```python
from build123d import *

# Parameters (mm, degrees)
SKETCH1_R           = 16
SKETCH1_R_2         = 12
BOSS_EXTRUDE1_DEPTH = 18
SKETCH1_3_R         = 3
BOSS_EXTRUDE2_DEPTH = 5
BOSS_EXTRUDE4_DEPTH = 18
SKETCH18_W          = 13
SKETCH18_H          = 2.498753947


with BuildPart() as part:
    # Sketch1 → Boss-Extrude1 (new body)
    with BuildSketch(Plane(origin=(0, 0, 0), x_dir=(1, 0, 0), z_dir=(0, 1, 0))):
        with Locations(Location((0, 0, 0), (0, 0, 270))):
            Circle(SKETCH1_R)
        with Locations(Location((0, 0, 0), (0, 0, 270))):
            Circle(SKETCH1_R_2, mode=Mode.SUBTRACT)
    extrude(amount=BOSS_EXTRUDE1_DEPTH)

    # Sketch1_3 → Boss-Extrude2 (add)
    with BuildSketch(Plane(origin=(0, 0, 0), x_dir=(1, 0, 0), z_dir=(0, 1, 0))):
        with BuildLine():
            ThreePointArc((-60, 32), (-64.242640687, 30.242640687), (-66, 26))
            Line((-66, 26), (-66, -26))
            ThreePointArc((-66, -26), (-64.242640687, -30.242640687), (-60, -32))
            Line((-60, -32), (60, -32))
            ThreePointArc((60, -32), (64.242640687, -30.242640687), (66, -26))
            Line((66, -26), (66, 26))
            ThreePointArc((66, 26), (64.242640687, 30.242640687), (60, 32))
            Line((60, 32), (-60, 32))
        make_face()
        with Locations(Location((-60, -26, 0), (0, 0, 270))):
            Circle(SKETCH1_3_R, mode=Mode.SUBTRACT)
        with Locations(Location((60, -26, 0), (0, 0, 270))):
            Circle(SKETCH1_3_R, mode=Mode.SUBTRACT)
        with Locations(Location((-60, 26, 0), (0, 0, 270))):
            Circle(SKETCH1_3_R, mode=Mode.SUBTRACT)
        with BuildLine():
            ThreePointArc((11.047086147, -11.574190583), (0, -16), (-11.047086147, -11.574190583))
            Line((-11.047086147, -11.574190583), (-36.72114317, -26.397114317))
            Line((-36.72114317, -26.397114317), (-41.22114317, -18.602885683))
            Line((-41.22114317, -18.602885683), (-15.547086147, -3.779961949))
            ThreePointArc((-15.547086147, -3.779961949), (-16, 0), (-15.547086147, 3.779961949))
            Line((-15.547086147, 3.779961949), (-41.22114317, 18.602885683))
            Line((-41.22114317, 18.602885683), (-36.72114317, 26.397114317))
            Line((-36.72114317, 26.397114317), (-11.047086147, 11.574190583))
            ThreePointArc((-11.047086147, 11.574190583), (0, 16), (11.047086147, 11.574190583))
            Line((11.047086147, 11.574190583), (36.72114317, 26.397114317))
            Line((36.72114317, 26.397114317), (41.22114317, 18.602885683))
            Line((41.22114317, 18.602885683), (15.547086147, 3.779961949))
            ThreePointArc((15.547086147, 3.779961949), (15.88636803, 1.903499625), (16, 0))
            ThreePointArc((16, 0), (15.88636803, -1.903499625), (15.547086147, -3.779961949))
            Line((15.547086147, -3.779961949), (41.22114317, -18.602885683))
            Line((41.22114317, -18.602885683), (36.72114317, -26.397114317))
            Line((36.72114317, -26.397114317), (11.047086147, -11.574190583))
        make_face(mode=Mode.SUBTRACT)
        with Locations(Location((60, 26, 0), (0, 0, 270))):
            Circle(SKETCH1_3_R, mode=Mode.SUBTRACT)
    extrude(amount=BOSS_EXTRUDE2_DEPTH)

    # Sketch1_6 → Boss-Extrude4 (add)
    with BuildSketch(Plane(origin=(0, 0, 0), x_dir=(1, 0, 0), z_dir=(0, 1, 0))):
        with BuildLine():
            Line((-41.22114317, 18.602885683), (-15.547086147, 3.779961949))
            ThreePointArc((-15.547086147, 3.779961949), (-13.856406461, 8), (-11.047086147, 11.574190583))
            Line((-11.047086147, 11.574190583), (-36.72114317, 26.397114317))
            Line((-36.72114317, 26.397114317), (-41.22114317, 18.602885683))
        make_face()
        with BuildLine():
            Line((36.72114317, 26.397114317), (11.047086147, 11.574190583))
            ThreePointArc((11.047086147, 11.574190583), (13.856406461, 8), (15.547086147, 3.779961949))
            Line((15.547086147, 3.779961949), (41.22114317, 18.602885683))
            Line((41.22114317, 18.602885683), (36.72114317, 26.397114317))
        make_face()
        with BuildLine():
            ThreePointArc((15.547086147, -3.779961949), (13.856406461, -8), (11.047086147, -11.574190583))
            Line((11.047086147, -11.574190583), (36.72114317, -26.397114317))
            Line((36.72114317, -26.397114317), (41.22114317, -18.602885683))
            Line((41.22114317, -18.602885683), (15.547086147, -3.779961949))
        make_face()
        with BuildLine():
            Line((-36.72114317, -26.397114317), (-11.047086147, -11.574190583))
            ThreePointArc((-11.047086147, -11.574190583), (-13.856406461, -8), (-15.547086147, -3.779961949))
            Line((-15.547086147, -3.779961949), (-41.22114317, -18.602885683))
            Line((-41.22114317, -18.602885683), (-36.72114317, -26.397114317))
        make_face()
    extrude(amount=BOSS_EXTRUDE4_DEPTH)

    # Sketch18 → Cut-Revolve4 (revolve, cut)
    with BuildSketch(Plane(origin=(0, 0, 0), x_dir=(0, -1, 0), z_dir=(-1, 0, 0)), mode=Mode.PRIVATE) as cut_revolve4_sk:
        Polygon((-18, 16), (-18, 45), (-5, 45), (-14.422671191, 16), align=None)
        with Locations((-11.5, 46.249376974)):
            Rectangle(SKETCH18_W, SKETCH18_H)
    revolve(cut_revolve4_sk.sketch.rotate(Axis((0, 18.9, 0), (0, -1, 0)), 223.665177219), axis=Axis((0, 18.9, 0), (0, -1, 0)), mode=Mode.SUBTRACT)


solid = part.part
```
Input: part model. Units: mm. Frame: model coordinates. A direction names the side the tool comes from. Coordinates: 2 decimals unless noted, no trailing zeros. Loops run counter-clockwise (first coordinate to the right, second up) from the corner with the lowest first, then second, coordinate; pieces in that order, holes last. Notation, with made-up numbers: M 32,29.5 L 80,29.5 A32 ccw 80,63.5 Z; hole C 45,79.5 d5. An arc over 180 degrees is marked long. Use a Markdown table: item, result. Add a question column.
1) Line query: L1, parallel to X at y = 3.15, z = 26; L2, parallel to Y at x = 54.5, z = 18; L3, parallel to Z at x = -6, y = 16. Output: solid intervals per line, ascending. Write a range as from..to.
2) Pin query (flat end, axial travel): P1, Ø1, axis at x = -44, z = -11, coming from the +Y side. Return the tip coordinate at first contact, or that it passes through.
3) Section D-D, the plane y = 16.5. Return the cut outline in (x, z), plus the area to 3 significant figures.
4) Set-up query: faces 1 (the flat face through (20.777, 8.598, 17.192)), 2 (the flat face through (14, 5, -15)), 3 (the flat face through (14, 0, 0)), 4 (the flat face through (-20.777, 8.598, -17.192)), 5 (the flat face through (25.63, 8.6, 9.6)). Return all of +Z, -Z, +X, -X, +Y, -Y with unobstructed straight access to the full face (end or side cutting, diameter ignored); none if empty.
5) Section C-C, the plane y = 8. Return the cut outline in (x, z), plus the area to 3 significant figures.
6) Draft query along Z for faces 6 (the conical face through (-23.501, 10.824, -13.444)), 7 (the flat face through (-21.134, 8.598, 17.398)), 8 (the flat face through (-25.63, 8.6, -9.6)). Return one class per face: +Z half, -Z half, draft (parallel to the pull), parting line (faces both ways), or undercut.
7) Section B-B, the plane x = 0. Return the cut outline in (y, z), plus the area to 3 significant figures.
8) Section A-A, the plane z = 0. Return the cut outline in (x, y), plus the area to 3 significant figures.
Answer below:
| question | item | result |
|---|---|---|
| 1 | L1 | -66..-63, -57..57, 63..66 |
| 1 | L2 | 0..5 |
| 1 | L3 | -14.83..-10.39, 10.39..14.83 |
| 2 | P1 | y = 5 |
| 3 | outline | C 0,0 d32; hole C 0,0 d24 |
| 3 | area | 352 mm2 |
| 4 | face 1 | +Z, +Y |
| 4 | face 2 | +Y |
| 4 | face 3 | +Z, -Z, +X, -X, -Y |
| 4 | face 4 | -Z, +Y |
| 4 | face 5 | +X, +Y |
| 5 | outline | M -32.98,-13.84 A35.77 ccw -28.48,-21.64 L -11.05,-11.57 A16 ccw 11.05,-11.57 L 28.48,-21.64 A35.77 ccw 32.98,-13.84 L 15.55,-3.78 A16 ccw 15.55,3.78 L 32.98,13.84 A35.77 ccw 28.48,21.64 L 11.05,11.57 A16 ccw -11.05,11.57 L -28.48,21.64 A35.77 ccw -32.98,13.84 L -15.55,3.78 A16 ccw -15.55,-3.78 Z; hole C 0,0 d24 |
| 5 | area | 1,070 mm2 |
| 6 | face 6 | -Z half |
| 6 | face 7 | +Z half |
| 6 | face 8 | undercut |
| 7 | outline | M 0,-32 L 5,-32 L 5,-16 L 18,-16 L 18,-12 L 0,-12 Z; M 0,12 L 18,12 L 18,16 L 5,16 L 5,32 L 0,32 Z |
| 7 | area | 304 mm2 |
| 8 | outline | M -66,0 L -12,0 L -12,18 L -16,18 L -16,5 L -66,5 Z; M 12,0 L 66,0 L 66,5 L 16,5 L 16,18 L 12,18 Z |
| 8 | area | 644 mm2 |
